Verification items for the finished model (mm, model axes). A direction names the side the tool comes from. Coordinates: 2 decimals unless noted, no trailing zeros. Order: outer loops, then holes, each group sorted by start corner. A loop starts at its lowest first (then second) coordinate and runs counter-clockwise, first axis right, second up. Notation, with made-up numbers: M -20,-34 L 32,-34 A21 cw 32,-4 Z; hole C 14.5,53.25 d4. An arc over 180 degrees is marked long. Return JSON: item names as keys, results as strings.
Autodesk Inventor part; units mm, degrees
ref_plane "YZ Plane" through (0, 0, 0) normal (1, 0, 0) x (0, 1, 0)
ref_plane "XZ Plane" through (0, 0, 0) normal (0, 1, 0) x (-1, 0, 0)
ref_plane "XY Plane" through (0, 0, 0) normal (0, 0, 1) x (1, 0, 0)
sketch "Sketch1" plane through (0, 0, 0) normal (0, 0, 1) x (1, 0, 0)
  line L0 (-8, 48) -> (8, 48)
  line L1 (8, 48) -> (8, -48)
  line L2 (8, -48) -> (-8, -48)
  line L3 (-8, -48) -> (-8, 48)
  point P0 (0, 0)
  dimension "d0" = 16
  dimension "d1" = 96
  dimension "d2" = 8
  dimension "d3" = 48
extrude "Extrusion1" add sketch "Sketch1" along normal blind 3.2
shell "Shell1" thickness 1.5 removed faces 1 at (-2.6667, 16, 0)
sketch "Sketch2" plane through (0, 0, 3.2) normal (0, 0, 1) x (1, 0, 0)
  circle A0 centre (4, -44) radius 2.5
  line L0 (8, 48) -> (8, -48)
  line L1 (8, -48) -> (-8, -48)
  dimension "d7" = 5
  dimension "d10" = 4
  dimension "d11" = 4
extrude "Extrusion2" add sketch "Sketch2" along normal blind 1.6
sketch "Sketch3" plane through (6.5, -46.5, 1.7) normal (0, 0, -1) x (-1, 0, 0)
  circle A0 centre (2.5, 2.5) radius 2.5
  circle A1 centre (2.5, 2.5) radius 1.2
  point P0 (6.5, 46.5)
  dimension "d18" = 2.4
extrude "Extrusion3" cut sketch "Sketch3" against normal blind 1.6 contours A1
pattern_linear "Rectangular Pattern1" count 12 spacing 8 along (0, 1, 0) count 2 spacing 8 along (-1, 0, 0) of "Extrusion2", "Extrusion3"
sketch "Sketch4" plane through (6.5, -46.5, 1.7) normal (0, 0, -1) x (-1, 0, 0)
  circle A0 centre (2.5, 10.5) radius 1.2
  circle A1 centre (2.5, 2.5) radius 1.2
  line L0 (0, 93) -> (0, 0)
  line L1 (0, 0) -> (13, 0)
  circle A2 centre (6.5, 6.5) radius 3.15
  circle A3 centre (6.5, 6.5) radius 2.5
  point P0 (6.5, 46.5)
  dimension "d21" = 6.5
  dimension "d22" = 6.5
  dimension "d23" = 10.5
  dimension "d24" = 2.5
  dimension "d25" = 5
  dimension "d26" = 6.3
extrude "Extrusion4" add sketch "Sketch4" along normal up to surface (1.7 mm away) contours A2
pattern_linear "Rectangular Pattern2" count 11 spacing 8 along (0, 1, 0) of "Extrusion4"
equation "\"d0\" = 0.8 * WIDTH"
equation "\"d1\" = 0.8 * LENGTH"
equation "\"d4\" = HEIGHT"
equation "\"d21\" = 0.5 * d23 + 0.5 * d24"
equation "\"d22\" = d21"
equation "\"WIDTH\" = 2"
equation "\"HEIGHT\" = 3.2"
properties part number "2445" material "Steel"
Q1. Draft check along Y on faces 4 (the face through (-4, 28, 3.3)), 5 (the face through (-7, 0, 0)). Enter one of: pulls with the +Y half, pulls with the -Y half, needs draft (parallel to the pull), parting line crosses it, or undercut.
Values:
{"face 4": "undercut", "face 5": "needs draft"}
Q2. Tool access check on faces 1 (the face through (3.67, -30.48, 3.99)), 2 (the face through (4, 4, 3.3)), 3 (the face through (4, -12, 4.8)). Record the directions out of +Z, -Z, +X, -X, +Y, -Y that give a thin tool (end or side, any length) a straight path to the whole face; none if there is none.
Values:
{"face 1": "+Z", "face 2": "-Z", "face 3": "+Z, +X, -X, +Y, -Y"}
Q3. Cross-section at B-B, the plane y = 24. Record the boundary of the cut face in (x, z).
Values:
{"outline": "M -8,0 L -6.5,0 L -6.5,1.7 L -3.15,1.7 L -3.15,0 L -2.5,0 L -2.5,1.7 L 2.5,1.7 L 2.5,0 L 3.15,0 L 3.15,1.7 L 6.5,1.7 L 6.5,0 L 8,0 L 8,3.2 L -8,3.2 Z"}
Q4. Cross-section at A-A, the plane y = -20. Record the boundary of the cut face in (x, z), and give its area (3 significant figures).
Values:
{"outline": "M -8,0 L -6.5,0 L -6.5,1.7 L -5.2,1.7 L -5.2,3.3 L -2.8,3.3 L -2.8,1.7 L 2.8,1.7 L 2.8,3.3 L 5.2,3.3 L 5.2,1.7 L 6.5,1.7 L 6.5,0 L 8,0 L 8,3.2 L 6.5,3.2 L 6.5,4.8 L 1.5,4.8 L 1.5,3.2 L -1.5,3.2 L -1.5,4.8 L -6.5,4.8 L -6.5,3.2 L -8,3.2 Z", "area": "37.4 mm^2"}
Q5. Go/stop test with flat-tipped pins: pin 1 (2.5 mm diameter, centred on x = 4, y = -44, fed in from -Z); pin 2 (0.7 mm diameter, centred on x = -4, y = 4, fed in from -Z); pin 3 (6 mm diameter, centred on x = 0, y = -16, fed in from +Z). Record where each tip stops, or that it passes through.
Values:
{"pin 1": "z = 1.7", "pin 2": "z = 3.3", "pin 3": "z = 3.2"}
Q6. Material ranges on line 1 along Y through (x, z) = (-5.5, 1.15); line 2 along X through (y, z) = (-9.5, 1.1); line 3 along X through (y, z) = (21, 1.8), recorded low to high.
Values:
{"line 1": "-48 to -46.5, 46.5 to 48", "line 2": "-8 to -6.5, -2.77 to -2, 2 to 2.77, 6.5 to 8", "line 3": "-8 to -4.66, -3.34 to 3.34, 4.66 to 8"}
